For this review, take the finished solid that the model builds, in its own axes (mm). A direction names the side the tool comes from. Round coordinates to 2 decimals unless told otherwise and drop trailing zeros. Order: outer loops, then holes, each group sorted by start corner. A loop starts at its lowest first (then second) coordinate and runs counter-clockwise, first axis right, second up. Notation, with made-up numbers: (64.5, 32.5) -> (83.5, 32.5) arc R33 ccw to (83.5, 63.5) -> close; hole circle Ø2 at (51.5, -27.75). An arc over 180 degrees is marked (long way). Use a Markdown table: item, result. Add a question column.
1) Consider section D-D (x = -27). State the section outline as (y, z) points.
2) Machinability: for faces 1 (the face through (9, -25, 2)), 2 (the face through (10.74, -12.32, -2.38)), which of the approach directions +Z, -Z, +X, -X, +Y, -Y give a long, thin tool a straight path to every point of the face, cutting with its end or side? Answer none if there is none.
3) Draft analysis for pull direction Z (two halves, no side actions). For faces 3 (the face through (-9, 3, -1)), 4 (the face through (2.703, -12.325, -8.584)), 5 (the face through (-17.235, 1.479, 41.569)), state which applies: pulls with the +Z half, pulls with the -Z half, needs draft (parallel to the pull), parting line crosses it, or undercut.
4) Wall thickness on line 1 along X through (y, z) = (-8.25, 0); line 2 along X through (y, z) = (2, 0); line 3 along Y through (x, z) = (19.5, -14): over which ranges is each line inside the solid? List them lowest first. Write a range as [from, to].
5) Consider section C-C (y = -11.5). State the section outline as (x, z) points.
6) Clearance check with flat-ended pins moving along their axes: P1, Ø3, axis at x = -24.5, z = -27, coming from the -Y side; P2, Ø14.5, axis at x = 0, z = 0, coming from the +Y side; P3, Ø1, axis at x = 0.5, y = -8.5, coming from the +Z side. State where each tip first meets the part, or that it passes through.
7) Consider section A-A (z = 0). State the section outline as (x, y) points, plus the area to 3 significant figures.
8) Consider section B-B (x = 0). State the section outline as (y, z) points, plus the area to 3 significant figures.
```python
from build123d import *

# Parameters (mm, degrees)
SKETCH1_R           = 45
SKETCH1_R_2         = 7.5
BOSS_EXTRUDE1_DEPTH = 3
SKETCH2_R           = 11
SKETCH2_R_2         = 9
BOSS_EXTRUDE2_DEPTH = 25


with BuildPart() as part:
    # Sketch1 → Boss-Extrude1 (new body)
    with BuildSketch(Plane(origin=(0, 0, 0), x_dir=(1, 0, 0), z_dir=(0, 1, 0))):
        with Locations(Location((0, 0, 0), (0, 0, 270))):
            Circle(SKETCH1_R)
        with Locations(Location((0, 0, 0), (0, 0, 270))):
            Circle(SKETCH1_R_2, mode=Mode.SUBTRACT)
    extrude(amount=BOSS_EXTRUDE1_DEPTH)

    # Sketch2 → Boss-Extrude2 (add)
    with BuildSketch(Plane.XZ):
        with Locations(Location((0, 0, 0), (0, 0, 90))):
            Circle(SKETCH2_R)
        with Locations(Location((0, 0, 0), (0, 0, 270))):
            Circle(SKETCH2_R_2, mode=Mode.SUBTRACT)
    extrude(amount=BOSS_EXTRUDE2_DEPTH)


solid = part.part
```
Results list:
| question | item | result |
|---|---|---|
| 1 | outline | (0, -36) -> (3, -36) -> (3, 36) -> (0, 36) -> close |
| 2 | face 1 | +Z, -Z, +X, -X, -Y |
| 2 | face 2 | -Y |
| 3 | face 3 | needs draft |
| 3 | face 4 | undercut |
| 3 | face 5 | parting line crosses it |
| 4 | line 1 | [-11, -9], [9, 11] |
| 4 | line 2 | [-45, -7.5], [7.5, 45] |
| 4 | line 3 | [0, 3] |
| 5 | outline | circle Ø22 at (0, 0); hole circle Ø18 at (0, 0) |
| 6 | P1 | y = 0 |
| 6 | P2 | through |
| 6 | P3 | z = 11 |
| 7 | outline | (-45, 0) -> (-11, 0) -> (-11, -25) -> (-9, -25) -> (-9, 0) -> (-7.5, 0) -> (-7.5, 3) -> (-45, 3) -> close; (7.5, 0) -> (9, 0) -> (9, -25) -> (11, -25) -> (11, 0) -> (45, 0) -> (45, 3) -> (7.5, 3) -> close |
| 7 | area | 325 mm2 |
| 8 | outline | (-25, -11) -> (0, -11) -> (0, -45) -> (3, -45) -> (3, -7.5) -> (0, -7.5) -> (0, -9) -> (-25, -9) -> close; (-25, 9) -> (0, 9) -> (0, 7.5) -> (3, 7.5) -> (3, 45) -> (0, 45) -> (0, 11) -> (-25, 11) -> close |
| 8 | area | 325 mm2 |
